```python
from build123d import *

# Parameters (mm, degrees)
EXTRUSION1_DEPTH = 3


with BuildPart() as part:
    # Esquisse1 → Extrusion1 (new body)
    with BuildSketch(Plane.XY):
        with BuildLine():
            Line((40.5, 232), (-40.5, 232))
            Line((-40.5, 232), (-40.5, 30))
            ThreePointArc((-40.5, 30), (-26.357864376, 24.142135624), (-20.5, 10))
            Line((-20.5, 10), (-20.5, 0))
            Line((-20.5, 0), (20.5, 0))
            Line((20.5, 0), (20.5, 10))
            ThreePointArc((20.5, 10), (26.357864376, 24.142135624), (40.5, 30))
            Line((40.5, 30), (40.5, 232))
        make_face()
    extrude(amount=EXTRUSION1_DEPTH)


solid = part.part
```
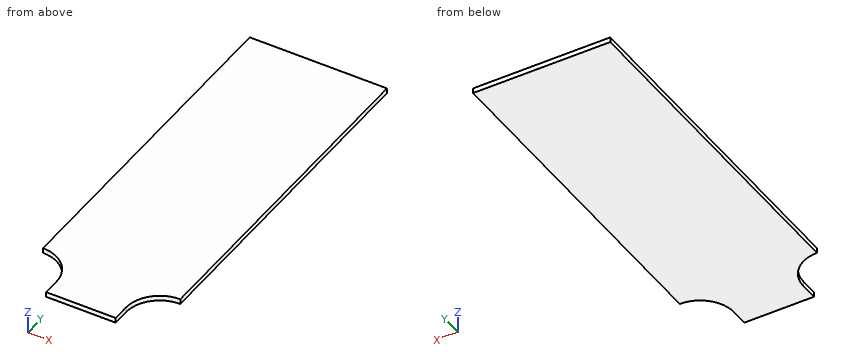
Here's how the part is built. I have some questions about the finished solid (model axes, mm). Coordinates: 2 decimals unless noted, no trailing zeros. Order: outer loops, then holes, each group sorted by start corner. A loop starts at its lowest first (then second) coordinate and runs counter-clockwise, first axis right, second up.
1) Imagine slicing it at A-A on z = 0.65. List the corners of the cut face in (x, y) for me, and give its area (3 significant figures).
2) Will this pin go through, and if not, where does the flat tip stop? pin 1 (1.5 mm diameter, centred on y = 7, z = 2, fed in from -X).
3) Imagine slicing it at B-B on y = 17. List the corners of the cut face in (x, z) for me (3 decimals).
4) Imagine slicing it at C-C on x = -29. List the corners of the cut face in (y, z) for me, and give its area (3 significant figures).
5) I need wall thicknesses on line 1 (X direction, y = 19.5, z = 1.9); line 2 (Y direction, x = 28.5, z = 0.75); line 3 (Y direction, x = -29.5, z = 1.4). Which ranges of each line are inside material? Lowest first, please.
Response values:
1. outline: (-40.5, 30) arc R20 cw to (-20.5, 10) - (-20.5, 0) - (20.5, 0) - (20.5, 10) arc R20 cw to (40.5, 30) - (40.5, 232) - (-40.5, 232) - close
1. area: 17,800 mm2
2. pin 1: stops at x = -20.5
3. outline: (-21.765, 0) - (21.765, 0) - (21.765, 3) - (-21.765, 3) - close
4. outline: (26.36, 0) - (232, 0) - (232, 3) - (26.36, 3) - close
4. area: 617 mm2
5. line 1: x = -22.9 to 22.9
5. line 2: y = 26 to 232
5. line 3: y = 26.7 to 232
